```python
from build123d import *

# Parameters (mm, degrees)
F0_R     = 2.5527
F0_R_2   = 14.2875
F1_DEPTH = 6.35
F2_R     = 76.2
F3_R     = 76.2
F4_W     = 30.394944
F4_H     = 7.431119
F4_W_2   = 30.836145
F4_H_2   = 7.137986
F5_DEPTH = 25.4


with BuildPart() as f1:
    # F0 (on Top) → F1 (new body)
    with BuildSketch(Plane.XY):
        with BuildLine():
            Line((-143.202675, -118.942378), (59.997325, -118.942378))
            ThreePointArc((59.997325, -118.942378), (88.261238, -65.278465), (34.597325, -93.542378))
            Line((34.597325, -93.542378), (-105.102675, -93.542378))
            Line((-105.102675, -93.542378), (-105.102675, 96.957622))
            Line((-105.102675, 96.957622), (34.597325, 96.957622))
            ThreePointArc((34.597325, 96.957622), (88.261238, 68.69371), (59.997325, 122.357622))
            Line((59.997325, 122.357622), (-143.202675, 122.357622))
            Line((-143.202675, 122.357622), (-143.202675, -118.942378))
        make_face()
        with Locations((48.284597, -105.255106)):
            Circle(F0_R, mode=Mode.SUBTRACT)
        with Locations((83.336597, -105.255106)):
            Circle(F0_R, mode=Mode.SUBTRACT)
        with Locations((65.810597, -87.729106)):
            Circle(F0_R_2, mode=Mode.SUBTRACT)
        with Locations((48.284597, -70.203106)):
            Circle(F0_R, mode=Mode.SUBTRACT)
        with Locations((83.336597, -70.203106)):
            Circle(F0_R, mode=Mode.SUBTRACT)
        with Locations((48.284597, 73.61835)):
            Circle(F0_R, mode=Mode.SUBTRACT)
        with Locations((65.810597, 91.14435)):
            Circle(F0_R_2, mode=Mode.SUBTRACT)
        with Locations((83.336597, 73.61835)):
            Circle(F0_R, mode=Mode.SUBTRACT)
        with Locations((48.284597, 108.67035)):
            Circle(F0_R, mode=Mode.SUBTRACT)
        with Locations((83.336597, 108.67035)):
            Circle(F0_R, mode=Mode.SUBTRACT)
    extrude(amount=F1_DEPTH)

    # F2
    f2_edges = [f1.edges().sort_by_distance(p)[0] for p in [
        (-105.102675, 96.957622, 3.175),
    ]]
    fillet(f2_edges, radius=F2_R)

    # F3
    f3_edges = [f1.edges().sort_by_distance(p)[0] for p in [
        (-105.102675, -93.542378, 3.175),
    ]]
    fillet(f3_edges, radius=F3_R)

    # F4 (on face) → F5 (cut)
    with BuildSketch(Plane.XY.offset(6.35)):
        with Locations((75.194797, 126.073181)):
            Rectangle(F4_W, F4_H)
        with Locations((75.415397, -122.511371)):
            Rectangle(F4_W_2, F4_H_2)
    extrude(amount=-F5_DEPTH, mode=Mode.SUBTRACT)


solid = f1.part
```
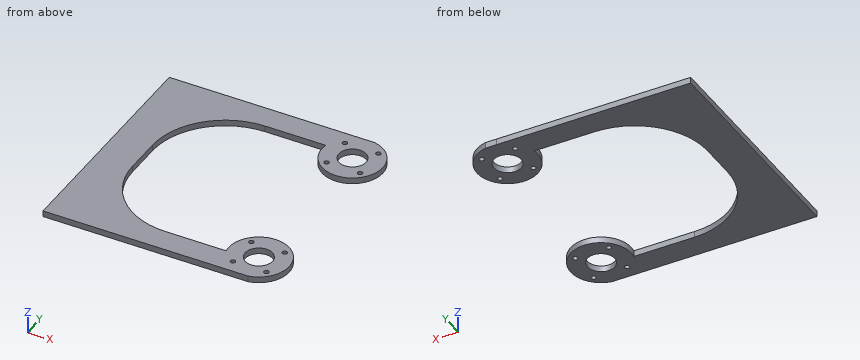
Here's how the part is built. I have some questions about the finished solid (model axes, mm). Round coordinates to 2 decimals unless told otherwise and drop trailing zeros. Order: outer loops, then holes, each group sorted by start corner. A loop starts at its lowest first (then second) coordinate and runs counter-clockwise, first axis right, second up. Notation, with made-up numbers: M -3,26.25 L 15,26.25 A12 cw 15,33.25 Z; hole C 75,-27.5 d6. An arc over 180 degrees is marked long. One line per question, with ' | ' between items.
1) I want a section at A-A, the plane x = -11.5. Write out the boundary of the cut face in (y, z).
Working result:
outline: M -118.94,0 L -93.54,0 L -93.54,6.35 L -118.94,6.35 Z; M 96.96,0 L 122.36,0 L 122.36,6.35 L 96.96,6.35 Z
2) I want a section at B-B, the plane y = -98. Write out the boundary of the cut face in (x, z), then the cut area to 3 significant figures.
Working result:
outline: M -143.2,0 L 55.88,0 L 55.88,6.35 L -143.2,6.35 Z; M 75.74,0 L 95.85,0 L 95.85,6.35 L 75.74,6.35 Z | area: 1,390 mm²
3) I want a section at D-D, the plane y = 81.5. Write out the boundary of the cut face in (x, z), then the cut area to 3 significant figures.
Working result:
outline: M -143.2,0 L -74.91,0 L -74.91,6.35 L -143.2,6.35 Z; M 35.56,0 L 55.27,0 L 55.27,6.35 L 35.56,6.35 Z; M 76.35,0 L 96.06,0 L 96.06,6.35 L 76.35,6.35 Z | area: 684 mm²
4) I need wall thicknesses on line 1 along X through (y, z) = (-80, 5.75); line 2 along Y through (x, z) = (-8.5, 1); line 3 along Y through (x, z) = (68.5, 3.75). Which ranges of each line are inside material? Lowest first, please.
Working result:
line 1: -143.2 to -72.27, 35.02 to 53.79, 77.83 to 96.61 | line 2: -118.94 to -93.54, 96.96 to 122.36 | line 3: -118.94 to -101.76, -73.7 to -56.09, 59.51 to 77.11, 105.18 to 122.36
5) I want a section at C-C, the plane z = 4.75. State how many separate pieces and enclosed holes the cut face has, then the cut area to 3 significant figures.
Working result:
separate pieces: 1 | enclosed holes: 10 | area: 24,000 mm²
6) For pin 1 Ø3 at (y, z) = (-82.5, 2) entering from +X; pin 2 Ø1.9 at (y, z) = (-5, 4) entering from +X; pin 3 Ø1 at (y, z) = (-39.5, 5) entering from +X, each with a flat end and sliding along its axis, tell me the tip position at first contact or that it passes through.
Working result:
pin 1: x = 97.34 | pin 2: x = -105.1 | pin 3: x = -101.66
